Build history of the part. All positions in model axes, mm. Face numbers are marked on the shaded views. A direction names the side the tool comes from. Coordinates: 2 decimals unless noted, no trailing zeros. Write each loop counter-clockwise with the first axis right and the second up, starting at its lowest first coordinate (ties: lowest second). Pieces come first, ordered by that corner, then holes.
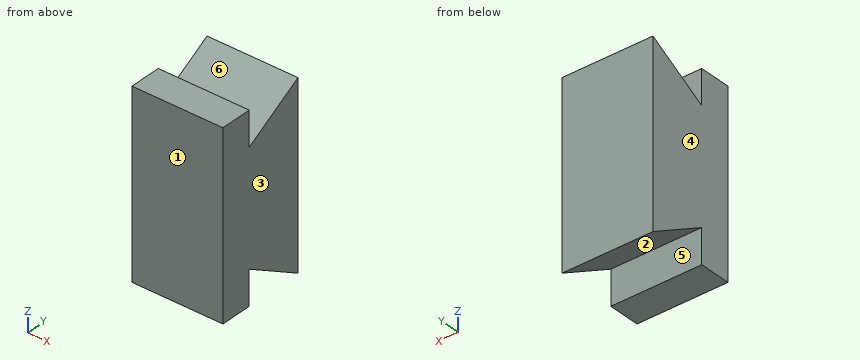
Autodesk Inventor part; units mm, degrees
ref_plane "YZ Plane" through (0, 0, 0) normal (1, 0, 0) x (0, 1, 0)
ref_plane "XZ Plane" through (0, 0, 0) normal (0, 1, 0) x (-1, 0, 0)
ref_plane "XY Plane" through (0, 0, 0) normal (0, 0, 1) x (1, 0, 0)
sketch "Sketch1" plane through (0, 0, 0) normal (1, 0, 0) x (0, 1, 0)
  line L0 (-7.5, -12.5) -> (7.5, -12.5)
  line L1 (7.5, -12.5) -> (7.5, 12.5)
  line L2 (7.5, 12.5) -> (-7.5, 12.5)
  line L3 (-7.5, 12.5) -> (-7.5, -12.5)
  line L4 (-7.5, -12.5) -> (7.5, 12.5) construction
  line L5 (7.5, -12.5) -> (-7.5, 12.5) construction
  point P0 (0, 0)
  dimension "d0" = 25
  dimension "d1" = 15
extrude "Extrusion1" add sketch "Sketch1" along normal blind 10
sketch "Sketch2" plane through (10, 0, 0) normal (1, 0, 0) x (0, 0, -1)
  line L0 (10, -7.5) -> (22, -7.5)
  line L1 (22, 12.5) -> (22, -7.5)
  line L2 (-35, 12.5) -> (22, 12.5)
  line L3 (-35, 12.5) -> (-35, 59.5)
  line L4 (-45, 59.5) -> (-35, 59.5)
  line L5 (-45, 59.5) -> (-45, -7.5)
  line L6 (-45, -7.5) -> (-10, -7.5)
  line L7 (-9.5, -7.5) -> (9.5, -7.5)
  line L8 (-10, -7.1) -> (-44.6, -7.1)
  line L9 (-44.6, -7.1) -> (-44.6, 59.1)
  line L10 (-44.6, 59.1) -> (-35.4, 59.1)
  line L11 (-35.4, 59.1) -> (-35.4, 12.1)
  line L12 (-35.4, 12.1) -> (21.6, 12.1)
  line L13 (21.6, 12.1) -> (21.6, -7.1)
  line L14 (21.6, -7.1) -> (10, -7.1)
  line L15 (10, -7.1) -> (10, -4)
  line L16 (10, -4) -> (6.2132, -4)
  line L17 (6.2132, -4) -> (9.966, 2.5)
  line L18 (9.966, 2.5) -> (-9.966, 2.5)
  line L19 (-9.966, 2.5) -> (-6.2132, -4)
  line L20 (-6.2132, -4) -> (-10, -4)
  line L21 (-10, -4) -> (-10, -7.1)
  line L22 (-10, -7.1) -> (-10, -7.5)
  line L23 (-12.5, -7.5) -> (12.5, -7.5)
  line L24 (10, -7.1) -> (10, -7.5)
  line L25 (-12.5, -7.5) -> (12.5, -7.5)
  circle A0 centre (-23.999, -0.85) radius 1.5
  line L26 (-10, -7.5) -> (-10, -4)
  line L27 (-10, -4) -> (-6.2132, -4)
  line L28 (-6.2132, -4) -> (-9.966, 2.5)
  line L29 (-9.966, 2.5) -> (9.966, 2.5)
  line L30 (9.966, 2.5) -> (6.2132, -4)
  line L31 (6.2132, -4) -> (10, -4)
  line L32 (10, -4) -> (10, -7.5)
  point P0 (0, 0)
extrude "Extrusion2" cut sketch "Sketch2" against normal blind 10 contours L24 L14 L13 L12 L11 L10 L9 L8 L22 L6 L5 L4 L3 L2 L1 L0 | L15 L16 L17 L18 L19 L20 L21 L8 L9 L10 L11 L12 L13 L14 | A0
properties part number "tester"
1. Saw through at D-D on y = -0.25. List the corners of the cut face in (x, z), plus the area to 3 significant figures.
Computed values:
outline: (0, -8.38) - (10, -8.38) - (10, 8.38) - (0, 8.38) - close
area: 168 mm2
2. Saw through at A-A on z = 6.75. List the corners of the cut face in (x, y), plus the area to 3 significant figures.
Computed values:
outline: (0, -7.5) - (10, -7.5) - (10, -4) - (0, -4) - close; (0, -3.07) - (10, -3.07) - (10, 2.5) - (0, 2.5) - close
area: 90.7 mm2
3. Probe line 1 along Y through (x, z) = (2.75, 8.25); line 2 along Y through (x, z) = (1, 9); line 3 along Z through (x, y) = (9.25, 0.5). List the from-to ranges inside material, lowest first.
Computed values:
line 1: y = -7.5 to -4, -0.47 to 2.5
line 2: y = -7.5 to -4, 0.83 to 2.5
line 3: z = -8.81 to 8.81
4. 3-axis set-ups, long thin cutter, end or side, ignore diameter. For the marked faces 4, 5 and 6: which of +Z, -Z, +X, -X, +Y, -Y reach the whole face in a straight line?
Computed values:
face 4: +Z, -Z, -X, +Y, -Y
face 5: -Z, +X, -X
face 6: +Z, +X, -X
5. Saw through at B-B on x = 4.5. List the corners of the cut face in (y, z).
Computed values:
outline: (-7.5, -10) - (-4, -10) - (-4, -6.21) - (2.5, -9.97) - (2.5, 9.97) - (-4, 6.21) - (-4, 10) - (-7.5, 10) - close
6. Saw through at C-C on y = 2. List the corners of the cut face in (x, z).
Computed values:
outline: (0, -9.68) - (10, -9.68) - (10, 9.68) - (0, 9.68) - close
7. Mould opens along Y. For the marked faces 1, 2 and 3 say: +Y half, -Y half, draft (parallel to the pull), parting line (faces both ways), or undercut.
Computed values:
face 1: -Y half
face 2: undercut
face 3: draft
8. Flat gauge pins, fed straight in: pin 1 (1 mm diameter, centred on x = 4, y = -2, fed in from -Z); pin 2 (1 mm diameter, centred on x = 4.5, y = 1, fed in from +Z); pin 3 (1.5 mm diameter, centred on x = 4.5, y = 1, fed in from -Z). Where does each tip first touch, or does it go through?
Computed values:
pin 1: stops at z = -7.66
pin 2: stops at z = 9.39
pin 3: stops at z = -9.53
